```python
from build123d import *

# Parameters (mm, degrees)
SKETCH2_W           = 12.5
SKETCH2_H           = 27
BOSS_EXTRUDE1_DEPTH = 28
SKETCH3_R           = 5
BOSS_EXTRUDE2_DEPTH = 4
SKETCH4_R           = 2.5
BOSS_EXTRUDE3_DEPTH = 5


with BuildPart() as part:
    # Sketch2 → Boss-Extrude1 (new body)
    with BuildSketch(Plane.XY):
        with Locations((6.25, 13.5)):
            Rectangle(SKETCH2_W, SKETCH2_H)
    extrude(amount=BOSS_EXTRUDE1_DEPTH)

    # Sketch3 → Boss-Extrude2 (add)
    with BuildSketch(Plane.XY.offset(28)):
        with Locations(Location((6.25, 7.381333163, 0), (0, 0, 180))):
            Circle(SKETCH3_R)
    extrude(amount=BOSS_EXTRUDE2_DEPTH)

    # Sketch4 → Boss-Extrude3 (add)
    with BuildSketch(Plane.XY.offset(32)):
        with Locations((6.25, 7.381333163)):
            Circle(SKETCH4_R)
    extrude(amount=BOSS_EXTRUDE3_DEPTH)


solid = part.part
```
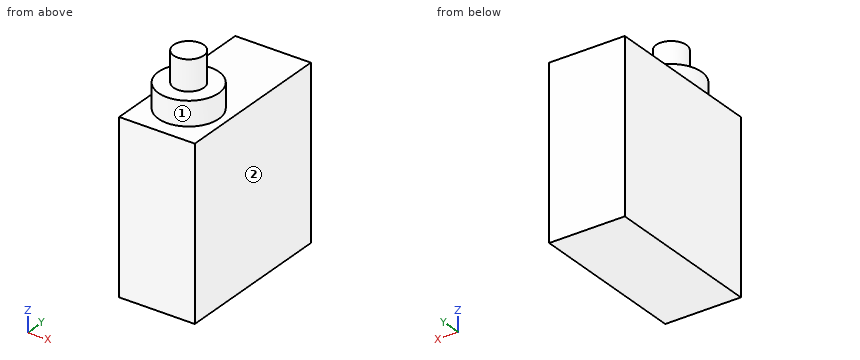
For this review, take the finished solid that the model builds, in its own axes (mm). Face numbers are marked on the shaded views. A direction names the side the tool comes from. Coordinates: 2 decimals unless noted, no trailing zeros. Write each loop counter-clockwise with the first axis right and the second up, starting at its lowest first coordinate (ties: lowest second). Pieces come first, ordered by that corner, then holes. Notation, with made-up numbers: (49.5, -39) - (70.5, -39) arc R34 cw to (70.5, -1) - close; hole circle Ø1 at (30.25, 3). An arc over 180 degrees is marked (long way). Put each result on its own line as item: value.
1. Add section D-D, the plane y = 21. Give the boundary of the cut face in (x, z).
Values found:
outline: (0, 0) - (12.5, 0) - (12.5, 28) - (0, 28) - close
2. Wall thickness on probe 1 along Z at (x, y) = (2.5, 2); probe 2 along Z at (x, y) = (7.5, 10); probe 3 along X at (y, z) = (6.5, 33): over which ranges is each line inside the solid? List them lowest first.
Values found:
probe 1: 0 to 28
probe 2: 0 to 32
probe 3: 3.91 to 8.59
3. Add section A-A, the plane x = 6.25. Give the boundary of the cut face in (y, z).
Values found:
outline: (0, 0) - (27, 0) - (27, 28) - (12.38, 28) - (12.38, 32) - (9.88, 32) - (9.88, 37) - (4.88, 37) - (4.88, 32) - (2.38, 32) - (2.38, 28) - (0, 28) - close
4. For pin 1 (1.5 mm diameter, centred on x = 2.5, y = 17, fed in from +Z), flat-tipped, find the tip position at first contact; note if it passes through.
Values found:
pin 1: z = 28
5. Machinability: for the marked faces 1 and 2, which of the approach directions +Z, -Z, +X, -X, +Y, -Y give a long, thin tool a straight path to every point of the face, cutting with its end or side? Answer none if there is none.
Values found:
face 1: +Z
face 2: +Z, -Z, +X, +Y, -Y
6. Add section C-C, the plane z = 33. Give the boundary of the cut face in (x, y), then the cut area to 3 significant figures.
Values found:
outline: circle Ø5 at (6.25, 7.38)
area: 19.6 mm²
7. Add section B-B, the plane y = 6.5. Give the boundary of the cut face in (x, z), then the cut area to 3 significant figures.
Values found:
outline: (0, 0) - (12.5, 0) - (12.5, 28) - (11.17, 28) - (11.17, 32) - (8.59, 32) - (8.59, 37) - (3.91, 37) - (3.91, 32) - (1.33, 32) - (1.33, 28) - (0, 28) - close
area: 413 mm²
